The figure shows three views and two pictorial views of one solid part (mm, origin at its lowest corner). Answer the questions. A direction names the side the tool comes from. Give positions to 0.01 mm unless a question says otherwise; leave off trailing zeros. Write each loop counter-clockwise with the first axis right and the second up, starting at its lowest first coordinate (ties: lowest second). Pieces come first, ordered by that corner, then holes. Notation, with made-up numbers: M 37.25,-19.5 L 45.25,-19.5 A24 cw 45.25,4.5 Z; hole C 37,-17 d7. An arc over 180 degrees is marked long. Answer as CSV lines item,"result". Start each with the question number.
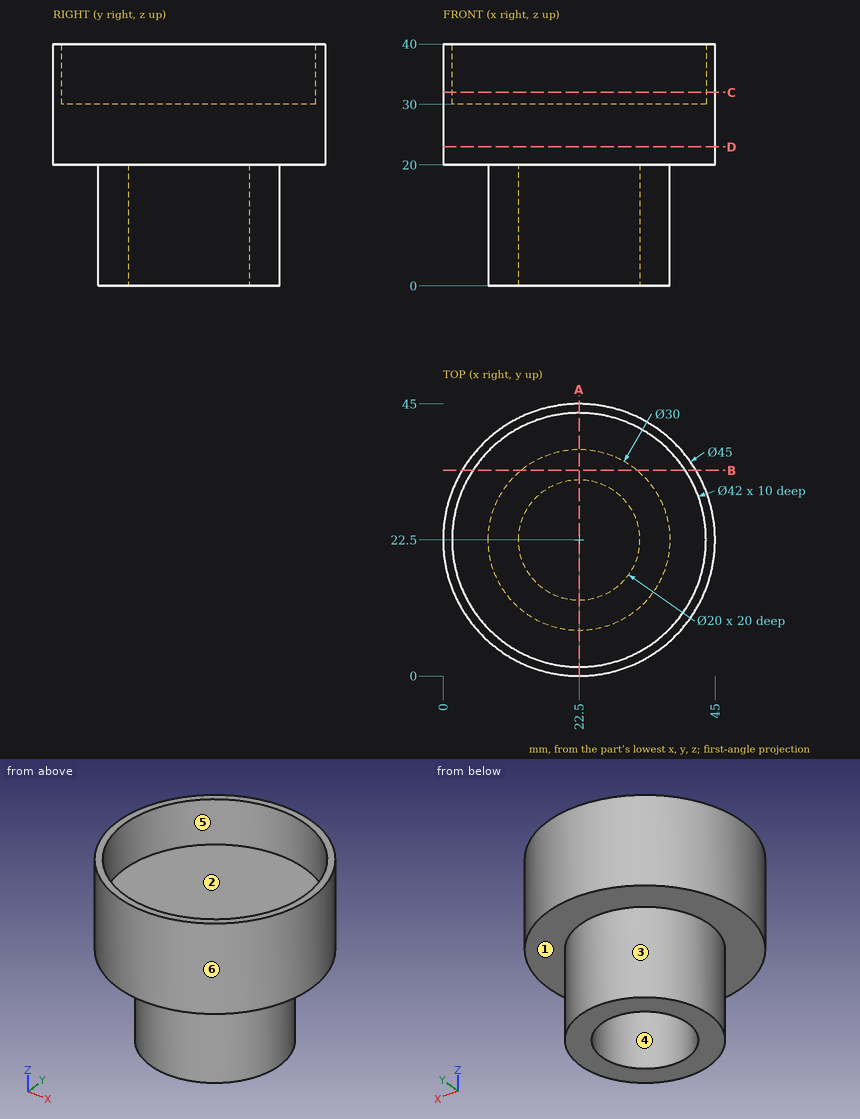
1. For the marked faces 5 and 6, determine the directions among +Z, -Z, +X, -X, +Y, -Y from which every point of the face is accessible in a straight line to the end or side of a thin tool.
2. Find the intervals of material crossed by line 1 (Y direction, x = 22, z = 37); line 2 (Y direction, x = 22, z = 14), in increasing order. Write a range as [from, to].
3. Find section C-C on z = 32. Determine the outline of the cut face in (x, y).
4. Given pin 1 (1 mm diameter, centred on y = 20, z = 29.5, fed in from -X); pin 2 (12 mm diameter, centred on y = 27.5, z = 14.5, fed in from +X); pin 3 (4 mm diameter, centred on x = 28, z = 22, fed in from +Y), each flat-ended and moving along its own axis, determine where each tip first touches the part or whether it passes through.
5. Determine the mould class of the marked faces 1, 2, 3 and 4 for opening direction Y: +Y half, -Y half, draft (parallel to the pull), parting line (faces both ways), or undercut.
6. Find section B-B on y = 34. Determine the outline of the cut face in (x, z), then the cut area to 3 significant figures.
7. Find section D-D on z = 23. Determine the outline of the cut face in (x, y), then the cut area to 3 significant figures.
8. Find section A-A on x = 22.5. Determine the outline of the cut face in (y, z).
Computed:
1,face 5,"+Z"
1,face 6,"+Z, -Z"
2,line 1,"y = [0.01, 1.51], [43.49, 44.99]"
2,line 2,"y = [7.51, 12.51], [32.49, 37.49]"
3,outline,"C 22.5,22.5 d45; hole C 22.5,22.5 d42"
4,pin 1,"stops at x = 0.09"
4,pin 2,"stops at x = 44.85"
4,pin 3,"stops at y = 44.73"
5,face 1,"draft"
5,face 2,"undercut"
5,face 3,"parting line"
5,face 4,"undercut"
6,outline,"M 3.16,20 L 12.87,20 L 12.87,0 L 32.13,0 L 32.13,20 L 41.84,20 L 41.84,40 L 40.07,40 L 40.07,30 L 4.93,30 L 4.93,40 L 3.16,40 Z"
6,area,"807 mm^2"
7,outline,"C 22.5,22.5 d45"
7,area,"1,590 mm^2"
8,outline,"M 0,20 L 7.5,20 L 7.5,0 L 12.5,0 L 12.5,20 L 32.5,20 L 32.5,0 L 37.5,0 L 37.5,20 L 45,20 L 45,40 L 43.5,40 L 43.5,30 L 1.5,30 L 1.5,40 L 0,40 Z"
